Autodesk Inventor part; units mm, degrees
ref_plane "YZ Plane" through (0, 0, 0) normal (1, 0, 0) x (0, 1, 0)
ref_plane "XZ Plane" through (0, 0, 0) normal (0, 1, 0) x (-1, 0, 0)
ref_plane "XY Plane" through (0, 0, 0) normal (0, 0, 1) x (1, 0, 0)
sketch "Sketch1" plane through (0, 0, 0) normal (0, 0, 1) x (1, 0, 0)
  line L0 (0, 0) -> (0, 10) construction
  line L1 (0, 0) -> (10, 0) construction
  line L2 (7.5, 5.5) -> (10, 5.5)
  line L3 (10, 5.5) -> (10, -5.5)
  line L4 (10, -5.5) -> (7.5, -5.5)
  line L5 (7.5, -5.5) -> (7.5, 5.5)
  line L6 (10, 5.2) -> (15.5, 5.2)
  line L7 (15.5, 5.2) -> (15.5, -5.2)
  line L8 (15.5, -5.2) -> (10, -5.2)
  line L9 (10, -5.2) -> (10, 5.2)
  line L10 (15.5, 5.5) -> (17.5, 5.5)
  line L11 (17.5, 5.5) -> (17.5, -5.5)
  line L12 (17.5, -5.5) -> (15.5, -5.5)
  line L13 (15.5, -5.5) -> (15.5, 5.5)
  dimension "d0" = 10
  dimension "d1" = 90
  dimension "d2" = 2.5
  dimension "d3" = 11
  dimension "d5" = 10.4
  dimension "d6" = 0.3
  dimension "d7" = 5.5
  dimension "d8" = 2
  dimension "d9" = 11
  dimension "d10" = 7.5
  dimension "d11" = 5.5
  dimension "d13" = 17.5
revolve "Revolution1" add sketch "Sketch1" angle 360 about axis through (0, 0, 0) along (0, 1, 0)
equation "\"d5\" = d9 - 2 * d6"
equation "\"d7\" = 0.5 * d3"
equation "\"d9\" = d3"
equation "\"d11\" = d7"
properties part number "6202-2rs_15x35x11" material "Steel"
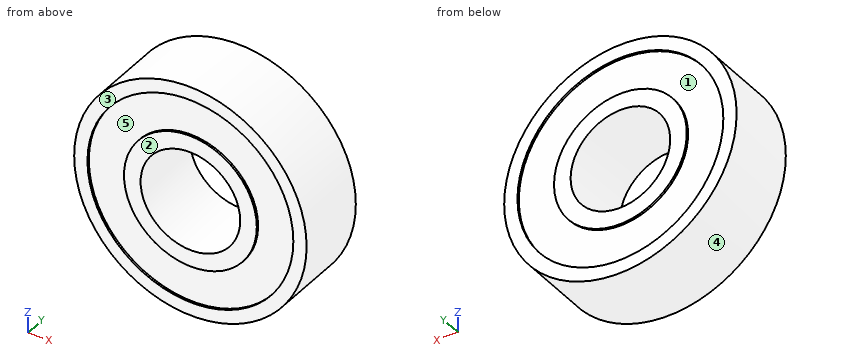
Geometry check sheet. Reference: the model listing, model coordinates, mm. Face numbers are marked on the shaded views. A direction names the side the tool comes from. Give positions to 0.01 mm unless a question says otherwise; leave off trailing zeros. Write each loop counter-clockwise with the first axis right and the second up, starting at its lowest first coordinate (ties: lowest second). Pieces come first, ordered by that corner, then holes.
1) Set-up check for the marked faces 1 and 2: record each of +Z, -Z, +X, -X, +Y, -Y from which the full face is reachable in a straight line by a thin tool's end or side.
Values follow:
face 1: +Y
face 2: +Z, -Z, +X, -X, -Y
2) Thickness scan on line 1 (X direction, y = 5.45, z = 0); line 2 (X direction, y = 3.25, z = 0). Record the ranges inside material, lowest first.
Values follow:
line 1: x = -17.5 to -15.5, -10 to -7.5, 7.5 to 10, 15.5 to 17.5
line 2: x = -17.5 to -7.5, 7.5 to 17.5
3) Cross-section at B-B (x = 0). Record the boundary of the cut face in (y, z), plus the area to 3 significant figures.
Values follow:
outline: (-5.5, -17.5) - (5.5, -17.5) - (5.5, -15.5) - (5.2, -15.5) - (5.2, -10) - (5.5, -10) - (5.5, -7.5) - (-5.5, -7.5) - (-5.5, -10) - (-5.2, -10) - (-5.2, -15.5) - (-5.5, -15.5) - close; (-5.5, 7.5) - (5.5, 7.5) - (5.5, 10) - (5.2, 10) - (5.2, 15.5) - (5.5, 15.5) - (5.5, 17.5) - (-5.5, 17.5) - (-5.5, 15.5) - (-5.2, 15.5) - (-5.2, 10) - (-5.5, 10) - close
area: 213 mm2
4) Go/stop test with flat-tipped pins: pin 1 Ø3 at (y, z) = (3, 10) entering from +X; pin 2 Ø3 at (y, z) = (1.5, 9) entering from -X; pin 3 Ø1.5 at (y, z) = (1, 6) entering from +X; pin 4 Ø8 at (x, z) = (-10, -9) entering from -Y. Record where each tip stops, or that it passes through.
Values follow:
pin 1: stops at x = 15.3
pin 2: stops at x = -15.81
pin 3: stops at x = 16.69
pin 4: stops at y = -5.5
5) Release check for a two-part mould opening along Z. For the marked faces 3, 4 and 5 record: released by +Z, released by -Z, zero draft, split by the parting line, or undercut.
Values follow:
face 3: zero draft
face 4: split by the parting line
face 5: undercut
6) Cross-section at D-D (z = 12). Record the boundary of the cut face in (x, y).
Values follow:
outline: (-12.74, -5.5) - (-9.81, -5.5) - (-9.81, -5.2) - (9.81, -5.2) - (9.81, -5.5) - (12.74, -5.5) - (12.74, 5.5) - (9.81, 5.5) - (9.81, 5.2) - (-9.81, 5.2) - (-9.81, 5.5) - (-12.74, 5.5) - close
7) Cross-section at C-C (y = -4.5). Record the boundary of the cut face in (x, z).
Values follow:
outline: circle Ø35 at (0, 0); hole circle Ø15 at (0, 0)
8) Cross-section at A-A (z = 0). Record the boundary of the cut face in (x, y), plus the area to 3 significant figures.
Values follow:
outline: (-17.5, -5.5) - (-15.5, -5.5) - (-15.5, -5.2) - (-10, -5.2) - (-10, -5.5) - (-7.5, -5.5) - (-7.5, 5.5) - (-10, 5.5) - (-10, 5.2) - (-15.5, 5.2) - (-15.5, 5.5) - (-17.5, 5.5) - close; (7.5, -5.5) - (10, -5.5) - (10, -5.2) - (15.5, -5.2) - (15.5, -5.5) - (17.5, -5.5) - (17.5, 5.5) - (15.5, 5.5) - (15.5, 5.2) - (10, 5.2) - (10, 5.5) - (7.5, 5.5) - close
area: 213 mm2
